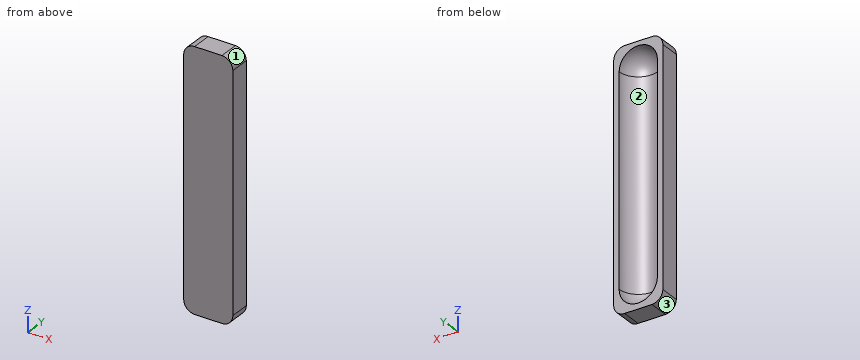
from build123d import *

# Parameters (mm, degrees)
SKETCH1_W           = 114.3
SKETCH1_H           = 596.9
BOSS_EXTRUDE1_DEPTH = 46.99
FILLET1_R           = 25.4


# Read off the part's stored shape, not the designer's step: Cut-Revolve1
with BuildPart() as part:
    # Sketch1 → Boss-Extrude1 (new body)
    with BuildSketch(Plane(origin=(0, 0, 0), x_dir=(1, 0, 0), z_dir=(0, 1, 0))):
        with Locations((-57.15, 298.45)):
            Rectangle(SKETCH1_W, SKETCH1_H)
    extrude(amount=BOSS_EXTRUDE1_DEPTH)

    # Cut-Revolve1 outline → Cut-Revolve1 (revolve, cut)
    with BuildSketch(Plane(origin=(-57.15, 46.99, 0), x_dir=(1, 0, 0), z_dir=(0, -1, 0))):
        with BuildLine():
            Line((0, -10.109470377), (0, -583.658766564))
            ThreePointArc((0, -583.658766564), (31.430896423, -570.639662987), (44.45, -539.208766564))
            Line((44.45, -539.208766564), (44.45, -54.559470377))
            ThreePointArc((44.45, -54.559470377), (31.430896424, -23.128573953), (0, -10.109470377))
        make_face()
    revolve(axis=Axis((-57.15, 46.99, 0), (0, 0, 1)), mode=Mode.SUBTRACT)

    # Fillet1
    fillet1_edges = [part.edges().sort_by_distance(p)[0] for p in [
        (-114.3, 23.495, -596.9),
        (0, 23.495, -596.9),
        (0, 23.495, 0),
        (-114.3, 23.495, 0),
    ]]
    fillet(fillet1_edges, radius=FILLET1_R)


solid = part.part
Build history of the part. All positions in model axes, mm. Face numbers are marked on the shaded views. Coordinates: 2 decimals unless noted, no trailing zeros. Write each loop counter-clockwise with the first axis right and the second up, starting at its lowest first coordinate (ties: lowest second). Pieces come first, ordered by that corner, then holes.
(1) Drill centre lines: line 1 (X direction, y = 35.5, z = -158); line 2 (X direction, y = 13.5, z = -327); line 3 (Z direction, x = -32.5, y = 22). Where is each one in solid material? Low to high.
(2) Pin check, flat tips, straight feed: pin 1 Ø12 at (x, z) = (-36.5, -301) entering from +Y (3 decimals); pin 2 Ø10 at (x, z) = (-63.5, -490.5) entering from -Y. Stop position of each tip, or through.
(3) Cut at D-D on x = -35.5. List the corners of the cut face in (y, z), and give its area (3 significant figures).
(4) Mould opens along Z. For the marked faces 1, 2 and 3 say: pulls with the +Z half, pulls with the -Z half, needs draft (parallel to the pull), parting line crosses it, or undercut.
(5) Cut at B-B on x = -57.15. List the corners of the cut face in (y, z).
(6) Cut at C-C on z = -135. List the corners of the cut face in (x, y).
(7) Cut at A-A on y = 8. List the corners of the cut face in (x, z), and give its area (3 significant figures).
Working result:
1. line 1: x = -114.3 to -100.09, -14.21 to 0
1. line 2: x = -114.3 to -86.38, -27.92 to 0
1. line 3: z = -596.9 to -566.48, -27.29 to 0
2. pin 1: stops at y = 11.415
2. pin 2: stops at y = 0
3. outline: (0, -596.9) - (46.99, -596.9) - (46.99, -578.03) arc R38.82 cw to (8.17, -539.21) - (8.17, -54.56) arc R38.82 cw to (46.99, -15.74) - (46.99, 0) - (0, 0) - close
3. area: 6,870 mm2
4. face 1: pulls with the +Z half
4. face 2: undercut
4. face 3: pulls with the -Z half
5. outline: (0, -596.9) - (46.99, -596.9) - (46.99, -583.66) arc R44.45 cw to (2.54, -539.21) - (2.54, -54.56) arc R44.45 cw to (46.99, -10.11) - (46.99, 0) - (0, 0) - close
6. outline: (-114.3, 0) - (0, 0) - (0, 46.99) - (-12.7, 46.99) arc R44.45 cw to (-101.6, 46.99) - (-114.3, 46.99) - close
7. outline: (-114.3, -571.5) arc R25.4 ccw to (-88.9, -596.9) - (-25.4, -596.9) arc R25.4 ccw to (0, -571.5) - (0, -25.4) arc R25.4 ccw to (-25.4, 0) - (-88.9, 0) arc R25.4 ccw to (-114.3, -25.4) - close; hole (-78.49, -539.21) arc R21.34 ccw to (-35.81, -539.21) - (-35.81, -54.56) arc R21.34 ccw to (-78.49, -54.56) - close
7. area: 45,600 mm2
